Build history of the part. All positions in model axes, mm. Round coordinates to 2 decimals unless told otherwise and drop trailing zeros. One line per question, with ' | ' between items.
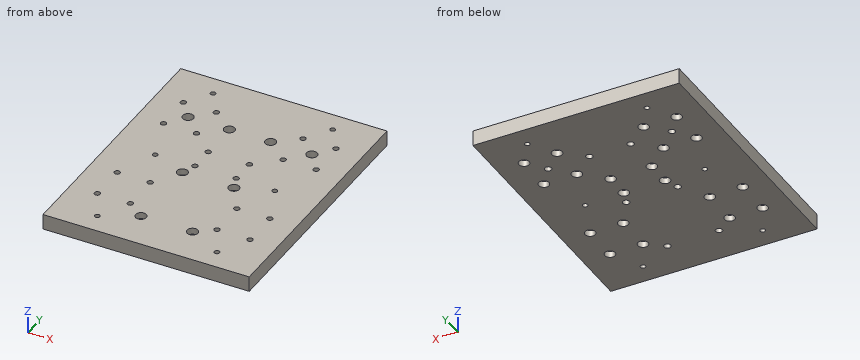
from build123d import *

# Parameters (mm, degrees)
SKETCH_W        = 200
SKETCH_H        = 250
PAD_DEPTH       = 15
SKETCH001_R     = 3.25
POCKET_DEPTH    = 15
SKETCH002_R     = 5.2
POCKET001_DEPTH = 6.2
SKETCH003_R     = 2.5
POCKET002_DEPTH = 15
SKETCH004_R     = 3.25
POCKET003_DEPTH = 15
SKETCH005_R     = 5.2
POCKET004_DEPTH = 7
SKETCH006_R     = 2.75
POCKET005_DEPTH = 15
SKETCH007_R     = 5
POCKET006_DEPTH = 6
SKETCH008_R     = 2.75
POCKET007_DEPTH = 15
SKETCH009_R     = 5
POCKET008_DEPTH = 6


with BuildPart() as part:
    # Sketch → Pad (new body)
    with BuildSketch(Plane.XY):
        with Locations((100, 125)):
            Rectangle(SKETCH_W, SKETCH_H)
    extrude(amount=PAD_DEPTH)

    # Sketch001 (on Face6 of Pad) → Pocket (cut)
    with BuildSketch(Plane.XY.offset(15)):
        with Locations((125, 37.5)):
            Circle(SKETCH001_R)
        with Locations((75, 37.5)):
            Circle(SKETCH001_R)
        with Locations((125, 112.5)):
            Circle(SKETCH001_R)
        with Locations((75, 112.5)):
            Circle(SKETCH001_R)
    extrude(amount=-POCKET_DEPTH, mode=Mode.SUBTRACT)

    # Sketch002 (on Face5 of Pocket) → Pocket001 (cut)
    with BuildSketch(Plane.XY.offset(15)):
        with Locations((75, 112.5)):
            Circle(SKETCH002_R)
        with Locations((125, 112.5)):
            Circle(SKETCH002_R)
        with Locations((75, 37.5)):
            Circle(SKETCH002_R)
        with Locations((125, 37.5)):
            Circle(SKETCH002_R)
    extrude(amount=-POCKET001_DEPTH, mode=Mode.SUBTRACT)

    # Sketch003 (on Face5 of Pocket001) → Pocket002 (cut)
    with BuildSketch(Plane.XY.offset(15)):
        with Locations((42, 230)):
            Circle(SKETCH003_R)
        with Locations((42, 125)):
            Circle(SKETCH003_R)
        with Locations((42, 20)):
            Circle(SKETCH003_R)
        with Locations((158, 230)):
            Circle(SKETCH003_R)
        with Locations((158, 125)):
            Circle(SKETCH003_R)
        with Locations((158, 20)):
            Circle(SKETCH003_R)
    extrude(amount=-POCKET002_DEPTH, mode=Mode.SUBTRACT)

    # Sketch004 (on Face5 of Pocket002) → Pocket003 (cut)
    with BuildSketch(Plane.XY.offset(15)):
        with Locations((40, 188.5)):
            Circle(SKETCH004_R)
        with Locations((80, 188.5)):
            Circle(SKETCH004_R)
        with Locations((120, 188.5)):
            Circle(SKETCH004_R)
        with Locations((160, 188.5)):
            Circle(SKETCH004_R)
    extrude(amount=-POCKET003_DEPTH, mode=Mode.SUBTRACT)

    # Sketch005 (on Face5 of Pocket003) → Pocket004 (cut)
    with BuildSketch(Plane.XY.offset(15)):
        with Locations((40, 188.5)):
            Circle(SKETCH005_R)
        with Locations((80, 188.5)):
            Circle(SKETCH005_R)
        with Locations((120, 188.5)):
            Circle(SKETCH005_R)
        with Locations((160, 188.5)):
            Circle(SKETCH005_R)
    extrude(amount=-POCKET004_DEPTH, mode=Mode.SUBTRACT)

    # Sketch006 (on Face5 of Pocket004) → Pocket005 (cut)
    with BuildSketch(Plane.XY.offset(15)):
        with Locations((26, 206)):
            Circle(SKETCH006_R)
        with Locations((58, 206)):
            Circle(SKETCH006_R)
        with Locations((26, 170)):
            Circle(SKETCH006_R)
        with Locations((58, 170)):
            Circle(SKETCH006_R)
        with Locations((26, 86)):
            Circle(SKETCH006_R)
        with Locations((58, 86)):
            Circle(SKETCH006_R)
        with Locations((26, 50)):
            Circle(SKETCH006_R)
        with Locations((58, 50)):
            Circle(SKETCH006_R)
        with Locations((142, 206)):
            Circle(SKETCH006_R)
        with Locations((174, 206)):
            Circle(SKETCH006_R)
        with Locations((142, 170)):
            Circle(SKETCH006_R)
        with Locations((174, 170)):
            Circle(SKETCH006_R)
        with Locations((142, 86)):
            Circle(SKETCH006_R)
        with Locations((174, 86)):
            Circle(SKETCH006_R)
        with Locations((142, 50)):
            Circle(SKETCH006_R)
        with Locations((174, 50)):
            Circle(SKETCH006_R)
    extrude(amount=-POCKET005_DEPTH, mode=Mode.SUBTRACT)

    # Sketch007 (on Face4 of Pocket005) → Pocket006 (cut)
    with BuildSketch(Plane(origin=(0, 0, 0), x_dir=(1, 0, 0), z_dir=(0, 0, -1))):
        with Locations((26, -50)):
            Circle(SKETCH007_R)
        with Locations((58, -50)):
            Circle(SKETCH007_R)
        with Locations((142, -50)):
            Circle(SKETCH007_R)
        with Locations((174, -50)):
            Circle(SKETCH007_R)
        with Locations((142, -86)):
            Circle(SKETCH007_R)
        with Locations((174, -86)):
            Circle(SKETCH007_R)
        with Locations((26, -86)):
            Circle(SKETCH007_R)
        with Locations((58, -86)):
            Circle(SKETCH007_R)
        with Locations((26, -170)):
            Circle(SKETCH007_R)
        with Locations((58, -170)):
            Circle(SKETCH007_R)
        with Locations((26, -206)):
            Circle(SKETCH007_R)
        with Locations((58, -206)):
            Circle(SKETCH007_R)
        with Locations((142, -170)):
            Circle(SKETCH007_R)
        with Locations((174, -170)):
            Circle(SKETCH007_R)
        with Locations((142, -206)):
            Circle(SKETCH007_R)
        with Locations((174, -206)):
            Circle(SKETCH007_R)
    extrude(amount=-POCKET006_DEPTH, mode=Mode.SUBTRACT)

    # Sketch008 (on Face5 of Pocket006) → Pocket007 (cut)
    with BuildSketch(Plane.XY.offset(15)):
        with Locations((80, 150)):
            Circle(SKETCH008_R)
        with Locations((120, 150)):
            Circle(SKETCH008_R)
        with Locations((80, 126)):
            Circle(SKETCH008_R)
        with Locations((120, 126)):
            Circle(SKETCH008_R)
    extrude(amount=-POCKET007_DEPTH, mode=Mode.SUBTRACT)

    # Sketch009 (on Face4 of Pocket007) → Pocket008 (cut)
    with BuildSketch(Plane(origin=(0, 0, 0), x_dir=(1, 0, 0), z_dir=(0, 0, -1))):
        with Locations((80, -126)):
            Circle(SKETCH009_R)
        with Locations((120, -126)):
            Circle(SKETCH009_R)
        with Locations((80, -150)):
            Circle(SKETCH009_R)
        with Locations((120, -150)):
            Circle(SKETCH009_R)
    extrude(amount=-POCKET008_DEPTH, mode=Mode.SUBTRACT)


solid = part.part
Q1. Saw through at A-A, the plane x = 58. State how many separate pieces and enclosed holes the cut face has, then the cut area to 3 significant figures.
Found:
separate pieces: 5 | enclosed holes: 0 | area: 3,310 mm^2
Q2. Drill centre lines: L1, parallel to Y at x = 58, z = 1.7; L2, parallel to X at y = 188.5, z = 2.5; L3, parallel to Y at x = 174, z = 13.25. Where is each one in solid material? Low to high. Write a range as from..to.
Found:
L1: 0..45, 55..81, 91..165, 175..201, 211..250 | L2: 0..36.75, 43.25..76.75, 83.25..116.75, 123.25..156.75, 163.25..200 | L3: 0..47.25, 52.75..83.25, 88.75..167.25, 172.75..203.25, 208.75..250
Q3. Drop flat-ended pins along their axis: pin 1 (11.5 mm diameter, centred on x = 74.5, y = 35, fed in from +Z); pin 2 (9 mm diameter, centred on x = 174, y = 170, fed in from -Z); pin 3 (8.5 mm diameter, centred on x = 75, y = 112.5, fed in from +Z). Give the stop position or say it passes through.
Found:
pin 1: z = 15 | pin 2: z = 6 | pin 3: z = 8.8
